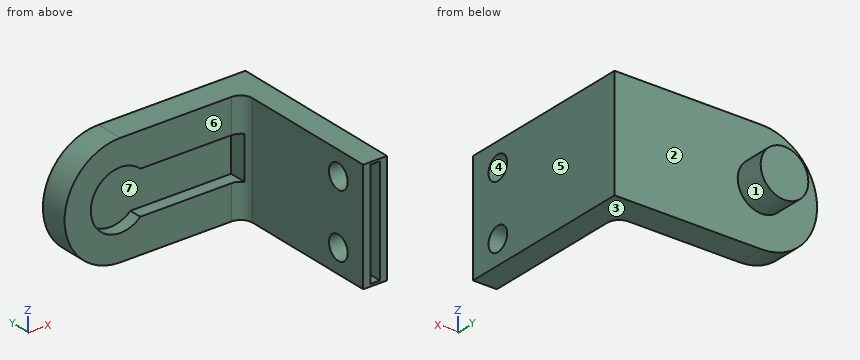
from build123d import *

# Parameters (mm, degrees)
BOSS_EXTRUDE1_DEPTH = 3.5
SKETCH2_W           = 3
SKETCH2_H           = 22.8
BOSS_EXTRUDE2_DEPTH = 7
SKETCH3_R           = 3
BOSS_EXTRUDE3_DEPTH = 3.7
SKETCH4_R           = 3.7
CUT_EXTRUDE2_DEPTH  = 1.6
CUT_EXTRUDE4_DEPTH  = 1.6
SKETCH6_W           = 1.2
SKETCH6_H           = 13.4
CUT_EXTRUDE6_DEPTH  = 2.2
SKETCH7_R           = 1.5
CUT_EXTRUDE7_DEPTH  = 3
FILLET1_R           = 1.5


with BuildPart() as part:
    # Sketch1 → Boss-Extrude1 (new body)
    with BuildSketch(Plane(origin=(0, 19.3, 0), x_dir=(1, 0, 0), z_dir=(0, 1, 0))):
        with BuildLine():
            Line((5.5, -7), (24, -7))
            Line((24, -7), (24, 7))
            Line((24, 7), (5.5, 7))
            ThreePointArc((5.5, 7), (-1.5, 0), (5.5, -7))
        make_face()
    extrude(amount=BOSS_EXTRUDE1_DEPTH)

    # Sketch2 → Boss-Extrude2 (add, symmetric)
    with BuildSketch(Plane.XY):
        with Locations((22.5, 11.4)):
            Rectangle(SKETCH2_W, SKETCH2_H)
    extrude(amount=BOSS_EXTRUDE2_DEPTH, both=True)

    # Sketch3 → Boss-Extrude3 (add)
    with BuildSketch(Plane(origin=(0, 22.8, 0), x_dir=(1, 0, 0), z_dir=(0, 1, 0))):
        with Locations(Location((5.5, 0, 0), (0, 0, 270))):
            Circle(SKETCH3_R)
    extrude(amount=BOSS_EXTRUDE3_DEPTH)

    # Sketch4 → Cut-Extrude2 (cut)
    with BuildSketch(Plane(origin=(0, 19.3, 0), x_dir=(1, 0, 0), z_dir=(0, 1, 0))):
        with Locations(Location((5.5, 0, 0), (0, 0, 270))):
            Circle(SKETCH4_R)
    extrude(amount=CUT_EXTRUDE2_DEPTH, mode=Mode.SUBTRACT)

    # Sketch5 → Cut-Extrude4 (cut)
    with BuildSketch(Plane(origin=(0, 19.3, 0), x_dir=(1, 0, 0), z_dir=(0, 1, 0))):
        with BuildLine():
            Line((5.5, -2.7), (20.7, -2.7))
            Line((20.7, -2.7), (20.7, 2.7))
            Line((20.7, 2.7), (5.5, 2.7))
            ThreePointArc((5.5, 2.7), (2.8, 0), (5.5, -2.7))
        make_face()
    extrude(amount=CUT_EXTRUDE4_DEPTH, mode=Mode.SUBTRACT)

    # Sketch6 → Cut-Extrude6 (cut)
    with BuildSketch(Plane(origin=(0, 0, 0), x_dir=(1, 0, 0), z_dir=(0, 1, 0))):
        with Locations((22.5, 0)):
            Rectangle(SKETCH6_W, SKETCH6_H)
    extrude(amount=CUT_EXTRUDE6_DEPTH, mode=Mode.SUBTRACT)

    # Sketch7 → Cut-Extrude7 (cut)
    with BuildSketch(Plane(origin=(24, 0, 0), x_dir=(0, 0, -1), z_dir=(1, 0, 0))):
        with Locations((-4, 4)):
            Circle(SKETCH7_R)
        with Locations((4, 4)):
            Circle(SKETCH7_R)
    extrude(amount=-CUT_EXTRUDE7_DEPTH, mode=Mode.SUBTRACT)

    # Fillet1
    # the kernel refuses this fillet: 1.5 mm, written as the material it adds along each edge
    with BuildSketch(Plane(origin=(21, 19.3, -7), x_dir=(-1, 0, 0), z_dir=(0, 0, 1))) as fillet1_piece_1_section:
        with BuildLine():
            CenterArc((FILLET1_R, FILLET1_R), FILLET1_R, 180, 90)
            Line((0, FILLET1_R), (0, 0))
            Line((0, 0), (FILLET1_R, 0))
        make_face()
    fillet1_piece_1 = extrude(amount=14, mode=Mode.PRIVATE)
    fillet1_piece_1 = split(fillet1_piece_1, bisect_by=Plane(origin=(20.368695353, 19.155022342, -2.7), z_dir=(0, 0, -1)), keep=Keep.TOP, mode=Mode.PRIVATE)
    fillet1_piece_1 = split(fillet1_piece_1, bisect_by=Plane(origin=(20.7, 19.155022342, -4.85), z_dir=(-1, 0, 0)), keep=Keep.TOP, mode=Mode.PRIVATE)
    add(fillet1_piece_1)
    with BuildSketch(Plane(origin=(21, 19.3, -7), x_dir=(-1, 0, 0), z_dir=(0, 0, 1))) as fillet1_piece_2_section:
        with BuildLine():
            CenterArc((FILLET1_R, FILLET1_R), FILLET1_R, 180, 90)
            Line((0, FILLET1_R), (0, 0))
            Line((0, 0), (FILLET1_R, 0))
        make_face()
    fillet1_piece_2 = extrude(amount=14, mode=Mode.PRIVATE)
    fillet1_piece_2 = split(fillet1_piece_2, bisect_by=Plane(origin=(20.890163131, 18.807126241, -2.7), z_dir=(0, 0, -1)), keep=Keep.TOP, mode=Mode.PRIVATE)
    fillet1_piece_2 = split(fillet1_piece_2, bisect_by=Plane(origin=(20.7, 18.807126241, -4.85), z_dir=(1, 0, 0)), keep=Keep.TOP, mode=Mode.PRIVATE)
    add(fillet1_piece_2)
    with BuildSketch(Plane(origin=(21, 19.3, -7), x_dir=(-1, 0, 0), z_dir=(0, 0, 1))) as fillet1_piece_3_section:
        with BuildLine():
            CenterArc((FILLET1_R, FILLET1_R), FILLET1_R, 180, 90)
            Line((0, FILLET1_R), (0, 0))
            Line((0, 0), (FILLET1_R, 0))
        make_face()
    fillet1_piece_3 = extrude(amount=14, mode=Mode.PRIVATE)
    fillet1_piece_3 = split(fillet1_piece_3, bisect_by=Plane(origin=(20.890163131, 18.807126241, 2.7), z_dir=(0, 0, -1)), keep=Keep.TOP, mode=Mode.PRIVATE)
    fillet1_piece_3 = split(fillet1_piece_3, bisect_by=Plane(origin=(20.890163131, 18.807126241, -2.7), z_dir=(0, 0, 1)), keep=Keep.TOP, mode=Mode.PRIVATE)
    fillet1_piece_3 = split(fillet1_piece_3, bisect_by=Plane(origin=(20.7, 18.807126241, 0), z_dir=(1, 0, 0)), keep=Keep.TOP, mode=Mode.PRIVATE)
    add(fillet1_piece_3)
    with BuildSketch(Plane(origin=(21, 19.3, -7), x_dir=(-1, 0, 0), z_dir=(0, 0, 1))) as fillet1_piece_4_section:
        with BuildLine():
            CenterArc((FILLET1_R, FILLET1_R), FILLET1_R, 180, 90)
            Line((0, FILLET1_R), (0, 0))
            Line((0, 0), (FILLET1_R, 0))
        make_face()
    fillet1_piece_4 = extrude(amount=14, mode=Mode.PRIVATE)
    fillet1_piece_4 = split(fillet1_piece_4, bisect_by=Plane(origin=(20.368695353, 19.155022342, 2.7), z_dir=(0, 0, 1)), keep=Keep.TOP, mode=Mode.PRIVATE)
    fillet1_piece_4 = split(fillet1_piece_4, bisect_by=Plane(origin=(20.7, 19.155022342, 4.85), z_dir=(-1, 0, 0)), keep=Keep.TOP, mode=Mode.PRIVATE)
    add(fillet1_piece_4)
    with BuildSketch(Plane(origin=(21, 19.3, -7), x_dir=(-1, 0, 0), z_dir=(0, 0, 1))) as fillet1_piece_5_section:
        with BuildLine():
            CenterArc((FILLET1_R, FILLET1_R), FILLET1_R, 180, 90)
            Line((0, FILLET1_R), (0, 0))
            Line((0, 0), (FILLET1_R, 0))
        make_face()
    fillet1_piece_5 = extrude(amount=14, mode=Mode.PRIVATE)
    fillet1_piece_5 = split(fillet1_piece_5, bisect_by=Plane(origin=(20.890163131, 18.807126241, 2.7), z_dir=(0, 0, 1)), keep=Keep.TOP, mode=Mode.PRIVATE)
    fillet1_piece_5 = split(fillet1_piece_5, bisect_by=Plane(origin=(20.7, 18.807126241, 4.85), z_dir=(1, 0, 0)), keep=Keep.TOP, mode=Mode.PRIVATE)
    add(fillet1_piece_5)


solid = part.part
Verification items for the finished model (mm, model axes). Face numbers are marked on the shaded views. A direction names the side the tool comes from. Coordinates: 2 decimals unless noted, no trailing zeros. Order: outer loops, then holes, each group sorted by start corner. A loop starts at its lowest first (then second) coordinate and runs counter-clockwise, first axis right, second up. Notation, with made-up numbers: M 27,70 L 55,70 A17 cw 55,88 Z; hole C 67.25,49.25 d1. An arc over 180 degrees is marked long. One line per item, written item: value. Start each with the question number.
Item 1: Thickness scan on probe 1 along Y at (x, z) = (22.9, 4); probe 2 along Z at (x, y) = (5.5, 19.65); probe 3 along Y at (x, z) = (0.25, 3). Record the ranges inside material, lowest first.
Item 2: Sectioned sample at B-B on z = 0. Record the cut outline in (x, y).
Item 3: Access from +Z, -Z, +X, -X, +Y, -Y to the whole of each face (thin tool, end or side, straight path). Record for the marked faces 5, 6 and 7.
Item 4: Sectioned sample at C-C on y = 13.5. Record the cut outline in (x, z), then the cut area to 3 significant figures.
Item 5: Sectioned sample at A-A on x = 9. Record the cut outline in (y, z), then the cut area to 3 significant figures.
Item 6: Depth check by flat-ended pin: P1, Ø1.5, axis at x = 3, z = -3, coming from the -Y side; P2, Ø6.5, axis at x = 5.5, z = 0, coming from the -Y side; P3, Ø0.7, axis at y = 1, z = 1, coming from the -X side. Enter the tip coordinate at first touch or a pass-through.
Item 7: Sectioned sample at D-D on x = 4.5. Record the cut outline in (y, z).
Item 8: Mould release check, pull along Z, two halves, no side actions. Record for the marked faces 1, 2, 3 and 4: pulls with the +Z half, pulls with the -Z half, needs draft (parallel to the pull), parting line crosses it, or undercut.
Calculated:
1. probe 1: 2.2 to 2.5, 5.5 to 22.8
1. probe 2: -7 to -3.7, 3.7 to 7
1. probe 3: 19.3 to 22.8
2. outline: M -1.5,19.3 L 1.8,19.3 L 1.8,20.9 L 20.7,20.9 L 20.7,18.7 A1.5 cw 21,17.8 L 21,0 L 21.9,0 L 21.9,2.2 L 23.1,2.2 L 23.1,0 L 24,0 L 24,22.8 L 8.5,22.8 L 8.5,26.5 L 2.5,26.5 L 2.5,22.8 L -1.5,22.8 Z
3. face 5: +Z, -Z, +X, +Y, -Y
3. face 6: +Z, -Z, -X, -Y
3. face 7: -Y
4. outline: M 21,-7 L 24,-7 L 24,7 L 21,7 Z
4. area: 42.0 mm^2
5. outline: M 19.3,-7 L 22.8,-7 L 22.8,7 L 19.3,7 L 19.3,2.7 L 20.9,2.7 L 20.9,-2.7 L 19.3,-2.7 Z
5. area: 40.4 mm^2
6. P1: y = 19.3
6. P2: y = 20.9
6. P3: x = 21
7. outline: M 19.3,-6.93 L 22.8,-6.93 L 22.8,-2.83 L 26.5,-2.83 L 26.5,2.83 L 22.8,2.83 L 22.8,6.93 L 19.3,6.93 L 19.3,3.56 L 20.9,3.56 L 20.9,-3.56 L 19.3,-3.56 Z
8. face 1: parting line crosses it
8. face 2: needs draft
8. face 3: pulls with the -Z half
8. face 4: undercut
